Autodesk Inventor part; units mm, degrees
ref_plane "YZ Plane" through (0, 0, 0) normal (1, 0, 0) x (0, 1, 0)
ref_plane "XZ Plane" through (0, 0, 0) normal (0, 1, 0) x (-1, 0, 0)
ref_plane "XY Plane" through (0, 0, 0) normal (0, 0, 1) x (1, 0, 0)
sketch "Skizze1" plane through (0, 0, 0) normal (1, 0, 0) x (0, 1, 0)
  line L0 (0, 0) -> (2.5, 0)
  line L1 (0, 0) -> (2.5, 0) construction
  line L2 (2.5, 0) -> (2.5, 7)
  line L3 (2.5, 7) -> (2, 7.5)
  line L4 (2, 7.5) -> (2, 8)
  line L5 (2, 8) -> (4, 8)
  line L6 (4, 8) -> (4, 88)
  line L7 (0, 93) -> (9.9588, 93)
  line L8 (9.9588, 93) -> (4, 88)
  line L9 (0, 0) -> (0, 93)
  line L10 (0, -18.6) -> (0, 111.6)
  dimension "d0" = 2.5
  dimension "d1" = 0
  dimension "d2" = 7
  dimension "d4" = 0.5
  dimension "d5" = 0.5
  dimension "d6" = 2
  dimension "d7" = 4
  dimension "d23" = 40
  dimension "d24" = 5
  dimension "d25" = 85
revolve "Umdrehung1" add sketch "Skizze1" angle 360 about axis through (0, 0, -10) along (0, 0, 1)
thread "Gewinde1"
shell "Wandung4" thickness 1 removed faces 1 at (-0.1358, 2.201, 93)
properties part number "Fuss1,0"
The model under review builds one solid part; all positions refer to its coordinate system, in mm. A direction names the side the tool comes from. Round coordinates to 2 decimals unless told otherwise and drop trailing zeros. Loops run counter-clockwise (first coordinate to the right, second up) from the corner with the lowest first, then second, coordinate; pieces in that order, holes last. Notation, with made-up numbers: (86, 76) - (138, 76) arc R15 cw to (138, 81) - close; hole circle Ø4 at (37, 81.5). An arc over 180 degrees is marked (long way). Write each question's results on one line, items separated by ' | '. Start each with the question number.
Q1. Take a section at A-A on y = 0. Give the boundary of the cut face in (x, z).
Q2. Wall thickness on line 1 along Y through (x, z) = (0, 30); line 2 along X through (y, z) = (0, 8.35); line 3 along Y through (x, z) = (0, 7.65): over which ranges is each line inside the solid? List them lowest first. Write a range as [from, to].
Q3. Draft analysis for pull direction X (two halves, no side actions). For faces 4 (the cylindrical face through (0, -3, 49)), 5 (the flat face through (1, -2, 8)), 6 (the cylindrical face through (3.905, -0.867, 48.56)), state which applies: pulls with the +X half, pulls with the -X half, needs draft (parallel to the pull), parting line crosses it, or undercut.
Q4. Insertion check: P1, Ø5, axis at x = 1, z = 70.5, coming from the -Y side; P2, Ø3, axis at x = -8, y = 6.5, coming from the +Z side; P3, Ø4, axis at x = -5.5, y = -5.5, coming from the -Z side; P4, Ø2, axis at x = 4.5, y = 7, coming from the -Z side. Each pin has a flat end and moves straight along its axis. Give the tip position at first contact, or say it passes through.
Q5. Take a section at C-C on z = 66.5. Give the boundary of the cut face in (x, y).
Q6. Tool access review of faces 1 (the cylindrical face through (1.952, -0.434, 7.754)), 2 (the cylindrical face through (2.44, -0.54, 3.55)), 3 (the cylindrical face through (1, 0, 8)): name each direction out of +Z, -Z, +X, -X, +Y, -Y from which nothing blocks a thin tool from reaching the whole face with its end or side.
Data:
1) outline: (-9.96, 93) - (-4, 88) - (-4, 8) - (-2, 8) - (-2, 7.5) - (-2.5, 7) - (-2.5, 0) - (2.5, 0) - (2.5, 7) - (2, 7.5) - (2, 8) - (4, 8) - (4, 88) - (9.96, 93) - (8.4, 93) - (3, 88.47) - (3, 9) - (1, 9) - (1, 7.09) - (1.5, 6.59) - (1.5, 1) - (-1.5, 1) - (-1.5, 6.59) - (-1, 7.09) - (-1, 9) - (-3, 9) - (-3, 88.47) - (-8.4, 93) - close
2) line 1: y = [-4, -3], [3, 4] | line 2: x = [-4, -1], [1, 4] | line 3: y = [-2, -1], [1, 2]
3) face 4: undercut | face 5: needs draft | face 6: parting line crosses it
4) P1: stops at y = -4 | P2: stops at z = 93 | P3: stops at z = 89.49 | P4: stops at z = 90.79
5) outline: circle Ø8 at (0, 0); hole circle Ø6 at (0, 0)
6) face 1: none | face 2: -Z | face 3: +Z
